Input: dimensioned drawing with shaded views. Units: mm. Origin: part minimum x, y, z. A direction names the side the tool comes from. Round coordinates to 2 decimals unless told otherwise and drop trailing zeros. Loops run counter-clockwise (first coordinate to the right, second up) from the corner with the lowest first, then second, coordinate; pieces in that order, holes last. Notation, with made-up numbers: M 83.5,16.25 L 128.5,16.25 A32 cw 128.5,44.25 Z; hole C 51.25,87.5 d3. An arc over 180 degrees is marked long. Put each result on its own line as item: value. Start each with the question number.
1) Reachability of the marked faces 1 and 2 from +Z, -Z, +X, -X, +Y, -Y: full face, straight path, thin tool, end or side. Return the list, or none.
2) Section A-A on x = 60. Output: boundary loops of the cut face in (y, z).
3) Section D-D on x = 15. Output: boundary loops of the cut face in (y, z), plus the area to 3 significant figures.
4) Pin query (flat end, axial travel): pin 1 (12 mm diameter, centred on x = 60, y = 58, fed in from -Z); pin 2 (2.5 mm diameter, centred on y = 59, z = 4, fed in from -X); pin 3 (3.5 mm diameter, centred on x = 60, y = 58, fed in from +Z). Return the tip coordinate at first contact, or that it passes through.
5) Line query: probe 1 along Y at (x, z) = (60, 3.25); probe 2 along Y at (x, z) = (60, 5.95); probe 3 along Y at (x, z) = (15, 5.25). Output: solid intervals per line, ascending.
6) Section C-C on y = 15. Output: boundary loops of the cut face in (x, z).
7) Section B-B on z = 3.5. Output: boundary loops of the cut face in (x, y), plus the area to 3 significant figures.
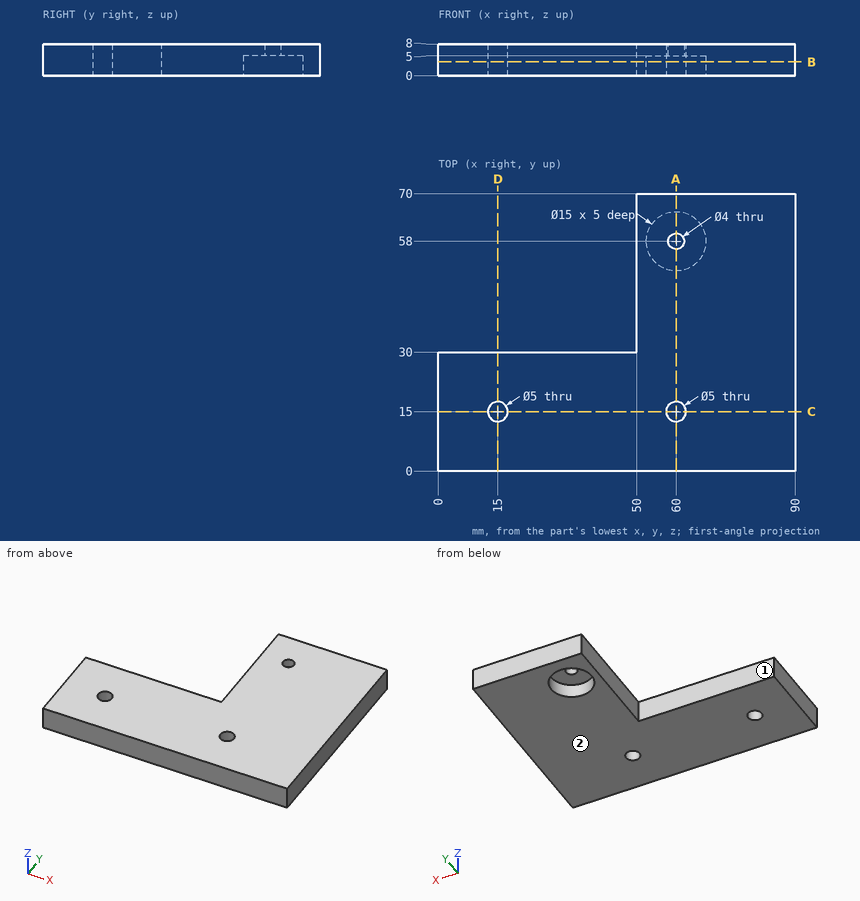
Geometry results:
1. face 1: +Z, -Z, -X, +Y
1. face 2: -Z, +X, -X, +Y, -Y
2. outline: M 0,0 L 12.5,0 L 12.5,8 L 0,8 Z; M 17.5,0 L 50.5,0 L 50.5,5 L 56,5 L 56,8 L 17.5,8 Z; M 60,5 L 65.5,5 L 65.5,0 L 70,0 L 70,8 L 60,8 Z
3. outline: M 0,0 L 12.5,0 L 12.5,8 L 0,8 Z; M 17.5,0 L 30,0 L 30,8 L 17.5,8 Z
3. area: 200 mm²
4. pin 1: stops at z = 5
4. pin 2: stops at x = 50
4. pin 3: passes through
5. probe 1: y = 0 to 12.5, 17.5 to 50.5, 65.5 to 70
5. probe 2: y = 0 to 12.5, 17.5 to 56, 60 to 70
5. probe 3: y = 0 to 12.5, 17.5 to 30
6. outline: M 0,0 L 12.5,0 L 12.5,8 L 0,8 Z; M 17.5,0 L 57.5,0 L 57.5,8 L 17.5,8 Z; M 62.5,0 L 90,0 L 90,8 L 62.5,8 Z
7. outline: M 0,0 L 90,0 L 90,70 L 50,70 L 50,30 L 0,30 Z; hole C 15,15 d5; hole C 60,58 d15; hole C 60,15 d5
7. area: 4,080 mm²
